```python
from build123d import *

# Parameters (mm, degrees)
ESQUISSE1_W             = 70
ESQUISSE1_H             = 26
BOSS_EXTRU_1_DEPTH      = 7
ESQUISSE2_W             = 8
ESQUISSE2_H             = 26
BOSS_EXTRU_2_DEPTH      = 45
BOSS_EXTRU_3_DEPTH      = 20
ENL_V_MAT_EXTRU_1_REACH = 89.184
ESQUISSE4_W             = 4
ESQUISSE4_H             = 20.5
CONG_1_R                = 1
CONG_2_R                = 2
ENL_V_MAT_EXTRU_2_REACH = 89.184
ESQUISSE5_R             = 1.6
CONG_3_R                = 6
ESQUISSE6_R             = 9.55
ENL_V_MAT_EXTRU_3_DEPTH = 6


with BuildPart() as part:
    # Esquisse1 → Boss.-Extru.1 (new body)
    with BuildSketch(Plane(origin=(0, 0, 0), x_dir=(1, 0, 0), z_dir=(0, 1, 0))):
        with Locations((35, 13)):
            Rectangle(ESQUISSE1_W, ESQUISSE1_H)
    extrude(amount=BOSS_EXTRU_1_DEPTH)

    # Esquisse2 → Boss.-Extru.2 (add)
    with BuildSketch(Plane(origin=(0, 7, 0), x_dir=(1, 0, 0), z_dir=(0, 1, 0))):
        with Locations((57, 13)):
            Rectangle(ESQUISSE2_W, ESQUISSE2_H)
    extrude(amount=BOSS_EXTRU_2_DEPTH)

    # Esquisse3 → Boss.-Extru.3 (add)
    with BuildSketch(Plane(origin=(0, 7, 0), x_dir=(1, 0, 0), z_dir=(0, 1, 0))):
        Polygon((53, 26), (12, 26), (12, 0), (53, 0), (53, 2.75), (14, 2.75), (14, 23.25), (53, 23.25), align=None)
    extrude(amount=BOSS_EXTRU_3_DEPTH)

    # Esquisse4 → Enlèv. mat.-Extru.1 (cut, up to next)
    with BuildSketch(Plane(origin=(0, 7, 0), x_dir=(1, 0, 0), z_dir=(0, 1, 0)), mode=Mode.PRIVATE) as enl_v_mat_extru_1_sk1:
        with Locations((25, 13)):
            Rectangle(ESQUISSE4_W, ESQUISSE4_H)
    enl_v_mat_extru_1_tool1 = extrude(enl_v_mat_extru_1_sk1.sketch, amount=-ENL_V_MAT_EXTRU_1_REACH, mode=Mode.PRIVATE) & part.part
    add(enl_v_mat_extru_1_tool1.solids().sort_by_distance((25, 7, -13))[0], mode=Mode.SUBTRACT)

    # Congé1
    cong_1_edges = [part.edges().sort_by_distance(p)[0] for p in [
        (53, 7, -13),
    ]]
    fillet(cong_1_edges, radius=CONG_1_R)

    # Congé2
    cong_2_edges = [part.edges().sort_by_distance(p)[0] for p in [
        (61, 7, -13),
        (12, 7, -13),
    ]]
    fillet(cong_2_edges, radius=CONG_2_R)

    # Esquisse5 → Enlèv. mat.-Extru.2 (cut, up to next)
    with BuildSketch(Plane(origin=(0, 7, 0), x_dir=(1, 0, 0), z_dir=(0, 1, 0)), mode=Mode.PRIVATE) as enl_v_mat_extru_2_sk1:
        with Locations(Location((6, 20, 0), (0, 0, 270))):
            Circle(ESQUISSE5_R)
    enl_v_mat_extru_2_tool1 = extrude(enl_v_mat_extru_2_sk1.sketch, amount=-ENL_V_MAT_EXTRU_2_REACH, mode=Mode.PRIVATE) & part.part
    # Esquisse5 → Enlèv. mat.-Extru.2 (cut, up to next)
    with BuildSketch(Plane(origin=(0, 7, 0), x_dir=(1, 0, 0), z_dir=(0, 1, 0)), mode=Mode.PRIVATE) as enl_v_mat_extru_2_sk2:
        with Locations(Location((66.5, 20, 0), (0, 0, 270))):
            Circle(ESQUISSE5_R)
    enl_v_mat_extru_2_tool2 = extrude(enl_v_mat_extru_2_sk2.sketch, amount=-ENL_V_MAT_EXTRU_2_REACH, mode=Mode.PRIVATE) & part.part
    # Esquisse5 → Enlèv. mat.-Extru.2 (cut, up to next)
    with BuildSketch(Plane(origin=(0, 7, 0), x_dir=(1, 0, 0), z_dir=(0, 1, 0)), mode=Mode.PRIVATE) as enl_v_mat_extru_2_sk3:
        with Locations(Location((66.5, 6, 0), (0, 0, 90))):
            Circle(ESQUISSE5_R)
    enl_v_mat_extru_2_tool3 = extrude(enl_v_mat_extru_2_sk3.sketch, amount=-ENL_V_MAT_EXTRU_2_REACH, mode=Mode.PRIVATE) & part.part
    # Esquisse5 → Enlèv. mat.-Extru.2 (cut, up to next)
    with BuildSketch(Plane(origin=(0, 7, 0), x_dir=(1, 0, 0), z_dir=(0, 1, 0)), mode=Mode.PRIVATE) as enl_v_mat_extru_2_sk4:
        with Locations(Location((6, 6, 0), (0, 0, 90))):
            Circle(ESQUISSE5_R)
    enl_v_mat_extru_2_tool4 = extrude(enl_v_mat_extru_2_sk4.sketch, amount=-ENL_V_MAT_EXTRU_2_REACH, mode=Mode.PRIVATE) & part.part
    add(enl_v_mat_extru_2_tool1.solids().sort_by_distance((6, 7, -20))[0], mode=Mode.SUBTRACT)
    add(enl_v_mat_extru_2_tool2.solids().sort_by_distance((66.5, 7, -20))[0], mode=Mode.SUBTRACT)
    add(enl_v_mat_extru_2_tool3.solids().sort_by_distance((66.5, 7, -6))[0], mode=Mode.SUBTRACT)
    add(enl_v_mat_extru_2_tool4.solids().sort_by_distance((6, 7, -6))[0], mode=Mode.SUBTRACT)

    # Congé3
    cong_3_edges = [part.edges().sort_by_distance(p)[0] for p in [
        (57, 52, -26),
        (57, 52, 0),
    ]]
    fillet(cong_3_edges, radius=CONG_3_R)

    # Esquisse6 → Enlèv. mat.-Extru.3 (cut)
    with BuildSketch(Plane(origin=(61, 0, 0), x_dir=(0, 0, -1), z_dir=(1, 0, 0))):
        with Locations((13, 38.53)):
            Circle(ESQUISSE6_R)
    extrude(amount=-ENL_V_MAT_EXTRU_3_DEPTH, mode=Mode.SUBTRACT)


solid = part.part
```
Geometry: final body of the model. Coordinates: model frame, mm. A direction names the side the tool comes from. Coordinates: 2 decimals unless noted, no trailing zeros. Loops run counter-clockwise (first coordinate to the right, second up) from the corner with the lowest first, then second, coordinate; pieces in that order, holes last. Notation, with made-up numbers: (74, 14.25) -> (128, 14.25) arc R12 ccw to (128, 29.25) -> close; hole circle Ø10 at (63, 49.25). An arc over 180 degrees is marked (long way). Use a Markdown table: item, result. Add a question column.
(1) Pin query (flat end, axial travel): pin 1 Ø14.5 at (y, z) = (17, -19.5) entering from -X; pin 2 Ø3 at (x, z) = (5.5, -12.5) entering from +Y; pin 3 Ø15.5 at (y, z) = (41.5, -15) entering from +X; pin 4 Ø1 at (x, y) = (43, 28.5) entering from +Z. Return the tip coordinate at first contact, or that it passes through.
(2) Section query D-D, the plane y = 21. Return loops of the section in (x, z).
(3) Section query C-C, the plane x = 66.5. Return loops of the section in (y, z), plus the area to 3 significant figures.
(4) Mould query, pull axis Z, two halves, no side actions, for faces 4 (the cylindrical face through (5.03, 3.55, -21.27)), 5 (the cylindrical face through (57.056, 50.289, -24.196)), 6 (the flat face through (5, 7, -13)). Classes: pulls with the +Z half, pulls with the -Z half, needs draft (parallel to the pull), parting line crosses it, or undercut.
(5) Section query A-A, the plane x = 57. Return loops of the section in (y, z).
(6) Access query for faces 1 (the flat face through (29, 27, -2)), 2 (the flat face through (33, 17, -2.75)), 3 (the flat face through (66, 7, -13)). Directions: +Z, -Z, +X, -X, +Y, -Y. A direction counts if a zero-diameter tool reaches every point of the face in a straight line with its end or side. Return the directions, or none.
(7) Section query B-B, the plane z = -17. Return loops of the section in (x, y).
(8) Line query: line 1 along X through (y, z) = (2, -6); line 2 along Z through (x, y) = (66.5, 4.75); line 3 along X through (y, z) = (14, -22). Output: solid intervals per line, ascending.
Answer:
| question | item | result |
|---|---|---|
| 1 | pin 1 | stops at x = 12 |
| 1 | pin 2 | stops at y = 7 |
| 1 | pin 3 | stops at x = 61 |
| 1 | pin 4 | passes through |
| 2 | outline | (12, -26) -> (61, -26) -> (61, 0) -> (12, 0) -> close; hole (14, -23.25) -> (53, -23.25) -> (53, -2.75) -> (14, -2.75) -> close |
| 3 | outline | (0, -26) -> (7, -26) -> (7, -21.6) -> (0, -21.6) -> close; (0, -18.4) -> (7, -18.4) -> (7, -7.6) -> (0, -7.6) -> close; (0, -4.4) -> (7, -4.4) -> (7, 0) -> (0, 0) -> close |
| 3 | area | 137 mm^2 |
| 4 | face 4 | undercut |
| 4 | face 5 | pulls with the -Z half |
| 4 | face 6 | needs draft |
| 5 | outline | (0, -26) -> (46, -26) arc R6 ccw to (52, -20) -> (52, -6) arc R6 ccw to (46, 0) -> (0, 0) -> close; hole circle Ø19.1 at (38.53, -13) |
| 6 | face 1 | +Z, -Z, -X, +Y |
| 6 | face 2 | +Y |
| 6 | face 3 | +Z, -Z, +X, +Y |
| 7 | outline | (0, 0) -> (23, 0) -> (23, 7) -> (14, 7) -> (14, 27) -> (12, 27) -> (12, 9) arc R2 cw to (10, 7) -> (0, 7) -> close; (27, 0) -> (70, 0) -> (70, 7) -> (63, 7) arc R2 cw to (61, 9) -> (61, 29.86) -> (55, 29.86) -> (55, 47.2) -> (61, 47.2) -> (61, 52) -> (53, 52) -> (53, 8) arc R1 cw to (52, 7) -> (27, 7) -> close |
| 8 | line 1 | x = 0 to 4.4, 7.6 to 23, 27 to 64.9, 68.1 to 70 |
| 8 | line 2 | z = -26 to -21.6, -18.4 to -7.6, -4.4 to 0 |
| 8 | line 3 | x = 12 to 14, 53 to 61 |
